Can you work these out from the model? Positions are in its coordinate system, mm. Face numbers are marked on the shaded views. A direction names the side the tool comes from. Coordinates: 2 decimals unless noted, no trailing zeros. Order: outer loops, then holes, each group sorted by start corner. A loop starts at its lowest first (then second) coordinate and runs counter-clockwise, first axis right, second up. Notation, with made-up numbers: (88, -39) -> (140, -39) arc R10 cw to (140, -30) -> close; hole circle Ø6 at (46, 31.25). An arc over 180 degrees is marked (long way). Answer in a Markdown table with one row per item. Add a question column.
1. Will these pins go through, and if not, where does the flat tip stop? pin 1 (1 mm diameter, centred on x = 3.5, z = 15, fed in from +Y); pin 2 (2.5 mm diameter, centred on x = -3.5, z = 3, fed in from -Y); pin 3 (4.5 mm diameter, centred on y = -3, z = 3.5, fed in from -X).
2. Imagine slicing it at B-B on y = -3. Write out the boundary of the cut face in (x, z), plus the area to 3 significant figures.
3. We'd pull the mould along Z, two halves only. Please class the marked faces 1, 2 and 3: pulls with the +Z half, pulls with the -Z half, needs draft (parallel to the pull), parting line crosses it, or undercut.
4. Imagine slicing it at D-D on z = 2.5. Write out the boundary of the cut face in (x, y).
5. If I drill on line 1 along Z through (x, y) = (-0.5, -6.5); line 2 along X through (y, z) = (-0.5, 3.5), over which ranges is the centre line in solid material (lowest first)? Write a range as [from, to].
6. Imagine slicing it at A-A on x = 0. Write out the boundary of the cut face in (y, z).
7. On a 3-axis mill with a long thin cutter (end or side, diameter ignored), from which of +Z, -Z, +X, -X, +Y, -Y can I reach the whole of each face in a straight line? I mean the marked faces 4, 5 and 6. Say none if no direction works.
8. Imagine slicing it at C-C on z = 8. Write out the boundary of the cut face in (x, y).
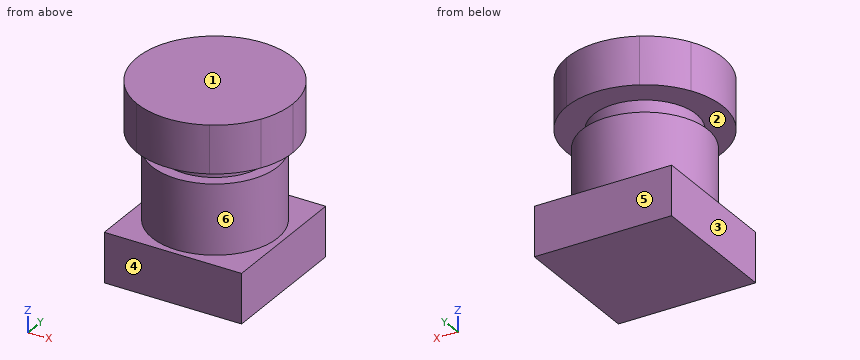
from build123d import *

# Parameters (mm, degrees)
F0_R     = 6.85
F0_R_2   = 5.6
F1_DEPTH = 5.4
F2_DEPTH = 13
F3_DEPTH = 15
F4_START = 15
F4_DEPTH = 5.21


with BuildPart() as f1:
    # F0 (on Top) → F1 (new body)
    with BuildSketch(Plane.XY):
        with BuildLine():
            ThreePointArc((4, 7.5), (6.0104076401, 6.0104076401), (7.5, 4))
            Line((7.5, 4), (7.5, 7.5))
            Line((7.5, 7.5), (4, 7.5))
        make_face()
        with BuildLine():
            Line((7.5, -4), (7.5, 4))
            ThreePointArc((7.5, 4), (6.0104076401, 6.0104076401), (4, 7.5))
            Line((4, 7.5), (-4, 7.5))
            ThreePointArc((-4, 7.5), (-6.0104076401, 6.0104076401), (-7.5, 4))
            Line((-7.5, 4), (-7.5, -4))
            ThreePointArc((-7.5, -4), (-6.0104076401, -6.0104076401), (-4, -7.5))
            Line((-4, -7.5), (4, -7.5))
            ThreePointArc((4, -7.5), (6.0104076401, -6.0104076401), (7.5, -4))
        make_face()
        Circle(F0_R, mode=Mode.SUBTRACT)
        Circle(F0_R)
        Circle(F0_R_2, mode=Mode.SUBTRACT)
        Circle(F0_R_2)
        with BuildLine():
            ThreePointArc((-7.5, 4), (-6.0104076401, 6.0104076401), (-4, 7.5))
            Line((-4, 7.5), (-7.5, 7.5))
            Line((-7.5, 7.5), (-7.5, 4))
        make_face()
        with BuildLine():
            Line((-7.5, -7.5), (-4, -7.5))
            ThreePointArc((-4, -7.5), (-6.0104076401, -6.0104076401), (-7.5, -4))
            Line((-7.5, -4), (-7.5, -7.5))
        make_face()
        with BuildLine():
            Line((7.5, -7.5), (7.5, -4))
            ThreePointArc((7.5, -4), (6.0104076401, -6.0104076401), (4, -7.5))
            Line((4, -7.5), (7.5, -7.5))
        make_face()
    extrude(amount=F1_DEPTH)

    # F0 (on Top) → F2 (join)
    with BuildSketch(Plane.XY):
        Circle(F0_R)
        Circle(F0_R_2, mode=Mode.SUBTRACT)
        Circle(F0_R_2)
    extrude(amount=F2_DEPTH)

    # F0 (on Top) → F3 (join)
    with BuildSketch(Plane.XY):
        Circle(F0_R_2)
    extrude(amount=F3_DEPTH)

    # F0 (on Top) → F4 (join)
    with BuildSketch(Plane.XY.offset(F4_START)):
        with BuildLine():
            Line((-7.5, -4), (-7.5, 4))
            ThreePointArc((-7.5, 4), (-8.5, 0), (-7.5, -4))
        make_face()
        with BuildLine():
            Line((7.5, -4), (7.5, 4))
            ThreePointArc((7.5, 4), (6.0104076401, 6.0104076401), (4, 7.5))
            Line((4, 7.5), (-4, 7.5))
            ThreePointArc((-4, 7.5), (-6.0104076401, 6.0104076401), (-7.5, 4))
            Line((-7.5, 4), (-7.5, -4))
            ThreePointArc((-7.5, -4), (-6.0104076401, -6.0104076401), (-4, -7.5))
            Line((-4, -7.5), (4, -7.5))
            ThreePointArc((4, -7.5), (6.0104076401, -6.0104076401), (7.5, -4))
        make_face()
        Circle(F0_R, mode=Mode.SUBTRACT)
        Circle(F0_R)
        Circle(F0_R_2, mode=Mode.SUBTRACT)
        Circle(F0_R_2)
        with BuildLine():
            ThreePointArc((-4, -7.5), (0, -8.5), (4, -7.5))
            Line((4, -7.5), (-4, -7.5))
        make_face()
        with BuildLine():
            ThreePointArc((7.5, -4), (8.2462112512, -2.0615528128), (8.5, 0))
            ThreePointArc((8.5, 0), (8.2462112512, 2.0615528128), (7.5, 4))
            Line((7.5, 4), (7.5, -4))
        make_face()
        with BuildLine():
            Line((-4, 7.5), (4, 7.5))
            ThreePointArc((4, 7.5), (0, 8.5), (-4, 7.5))
        make_face()
    extrude(amount=F4_DEPTH)


solid = f1.part
Answers follow:
| question | item | result |
|---|---|---|
| 1 | pin 1 | stops at y = 7.95 |
| 1 | pin 2 | stops at y = -7.5 |
| 1 | pin 3 | stops at x = -7.5 |
| 2 | outline | (-7.95, 15) -> (-4.73, 15) -> (-4.73, 13) -> (-6.16, 13) -> (-6.16, 5.4) -> (-7.5, 5.4) -> (-7.5, 0) -> (7.5, 0) -> (7.5, 5.4) -> (6.16, 5.4) -> (6.16, 13) -> (4.73, 13) -> (4.73, 15) -> (7.95, 15) -> (7.95, 20.21) -> (-7.95, 20.21) -> close |
| 2 | area | 276 mm² |
| 3 | face 1 | pulls with the +Z half |
| 3 | face 2 | undercut |
| 3 | face 3 | needs draft |
| 4 | outline | (-7.5, -7.5) -> (7.5, -7.5) -> (7.5, 7.5) -> (-7.5, 7.5) -> close |
| 5 | line 1 | z = [0, 13], [15, 20.21] |
| 5 | line 2 | x = [-7.5, 7.5] |
| 6 | outline | (-8.5, 15) -> (-5.6, 15) -> (-5.6, 13) -> (-6.85, 13) -> (-6.85, 5.4) -> (-7.5, 5.4) -> (-7.5, 0) -> (7.5, 0) -> (7.5, 5.4) -> (6.85, 5.4) -> (6.85, 13) -> (5.6, 13) -> (5.6, 15) -> (8.5, 15) -> (8.5, 20.21) -> (-8.5, 20.21) -> close |
| 7 | face 4 | -Z, +X, -X, -Y |
| 7 | face 5 | -Z, +X, -X, +Y |
| 7 | face 6 | none |
| 8 | outline | circle Ø13.7 at (0, 0) |
